Here's how the part is built. I have some questions about the finished solid (model axes, mm). A direction names the side the tool comes from. Give positions to 0.01 mm unless a question says otherwise; leave off trailing zeros. Loops run counter-clockwise (first coordinate to the right, second up) from the corner with the lowest first, then second, coordinate; pieces in that order, holes last. Notation, with made-up numbers: (-11, -28) - (8, -28) arc R11 cw to (8, -8) - close; hole circle Ø10 at (-34.75, 70.25). An arc over 180 degrees is marked (long way). Use one line per item in the form item = value.
from build123d import *

# Parameters (mm, degrees)
BOSS_EXTRUDE1_DEPTH = 3.1
SKETCH2_R           = 2.475
BOSS_EXTRUDE2_DEPTH = 2
CUT_EXTRUDE1_DEPTH  = 2


with BuildPart() as part:
    # Sketch1 → Boss-Extrude1 (new body)
    with BuildSketch(Plane(origin=(0, 0, 0), x_dir=(1, 0, 0), z_dir=(0, 1, 0))):
        Polygon((0, 0), (7.95, 0), (7.95, -7.95), (15.9, -7.95), (15.9, -15.9), (0, -15.9), align=None)
    extrude(amount=BOSS_EXTRUDE1_DEPTH)

    # Sketch2 → Boss-Extrude2 (add)
    with BuildSketch(Plane(origin=(0, 3.1, 0), x_dir=(1, 0, 0), z_dir=(0, 1, 0))):
        with Locations(Location((3.975, -3.975, 0), (0, 0, 270))):
            Circle(SKETCH2_R)
        with Locations(Location((3.975, -11.925, 0), (0, 0, 270))):
            Circle(SKETCH2_R)
        with Locations(Location((11.925, -11.925, 0), (0, 0, 270))):
            Circle(SKETCH2_R)
    extrude(amount=BOSS_EXTRUDE2_DEPTH)

    # Sketch3 → Cut-Extrude1 (cut)
    with BuildSketch(Plane.XZ):
        Polygon((1.5, 14.4), (1.5, 1.5), (6.45, 1.5), (6.45, 9.45), (14.4, 9.45), (14.4, 14.4), align=None)
    extrude(amount=-CUT_EXTRUDE1_DEPTH, mode=Mode.SUBTRACT)


solid = part.part
(1) For faces 4 (the cylindrical face through (4.718, 4.086, 14.286)), 5 (the flat face through (14.4, 1, 12)), 6 (the flat face through (8, 2, 15.9)), 7 (the flat face through (12, 2, 7.95)), which set-ups out of +Z, -Z, +X, -X, +Y, -Y let a thin tool reach every point of the face, with its end or its side?
Geometry says:
face_4 = +Y
face_5 = -Y
face_6 = +Z, +X, -X, +Y, -Y
face_7 = -Z, +X, +Y, -Y
(2) If we section it at C-C (z = 5): List the corners of the cut face in (x, y) for me, plus the area to 3 significant figures.
Geometry says:
outline = (0, 0) - (1.5, 0) - (1.5, 2) - (6.45, 2) - (6.45, 0) - (7.95, 0) - (7.95, 3.1) - (6.23, 3.1) - (6.23, 5.1) - (1.72, 5.1) - (1.72, 3.1) - (0, 3.1) - close
area = 23.8 mm²
(3) For P1, Ø3, axis at x = 8, z = 12.5, coming from the -Y side; P2, Ø0.9, axis at y = 1, z = 4, coming from the +X side; P3, Ø0.6, axis at x = 11, y = 1, coming from the -Z side, each with a flat end and sliding along its axis, tell me the tip position at first contact or that it passes through.
Geometry says:
P1 = 2
P2 = 7.95
P3 = 7.95
(4) If we section it at A-A (y = 0.4): List the corners of the cut face in (x, z) for me, plus the area to 3 significant figures.
Geometry says:
outline = (0, 0) - (7.95, 0) - (7.95, 7.95) - (15.9, 7.95) - (15.9, 15.9) - (0, 15.9) - close; hole (1.5, 1.5) - (6.45, 1.5) - (6.45, 9.45) - (14.4, 9.45) - (14.4, 14.4) - (1.5, 14.4) - close
area = 86.4 mm²
(5) If we section it at D-D (y = 2.9): List the corners of the cut face in (x, z) for me, plus the area to 3 significant figures.
Geometry says:
outline = (0, 0) - (7.95, 0) - (7.95, 7.95) - (15.9, 7.95) - (15.9, 15.9) - (0, 15.9) - close
area = 190 mm²
(6) Thinking about a two-plate mould opening in X: for faces 1 (the flat face through (7.95, 2, 4)), 2 (the flat face through (4, 5.1, 4)), 3 (the flat face through (10, 1, 9.45)), which applies, pulls with the +X half, pulls with the -X half, needs draft (parallel to the pull), parting line crosses it, or undercut?
Geometry says:
face_1 = pulls with the +X half
face_2 = needs draft
face_3 = undercut
(7) If I drill on probe 1 along X at (y, z) = (1.3, 10.5); probe 2 along X at (y, z) = (1, 8.25), over which ranges is the centre line in solid material (lowest first)?
Geometry says:
probe_1 = 0 to 1.5, 14.4 to 15.9
probe_2 = 0 to 1.5, 6.45 to 15.9
(8) If we section it at B-B (x = 7.5): List the corners of the cut face in (y, z) for me.
Geometry says:
outline = (0, 0) - (3.1, 0) - (3.1, 15.9) - (0, 15.9) - (0, 14.4) - (2, 14.4) - (2, 9.45) - (0, 9.45) - close
